Verification items for this drawing (mm, ordinates from the low corner). Give positions to 0.01 mm unless a question says otherwise; leave off trailing zeros. Loops run counter-clockwise (first coordinate to the right, second up) from the corner with the lowest first, then second, coordinate; pieces in that order, holes last. Notation, with made-up numbers: M 30.25,49.25 L 89.25,49.25 A16 ccw 89.25,70.25 Z; hole C 58.25,-30.5 d5. An arc over 180 degrees is marked long. Put each result on its own line as item: value. Start each with the question number.
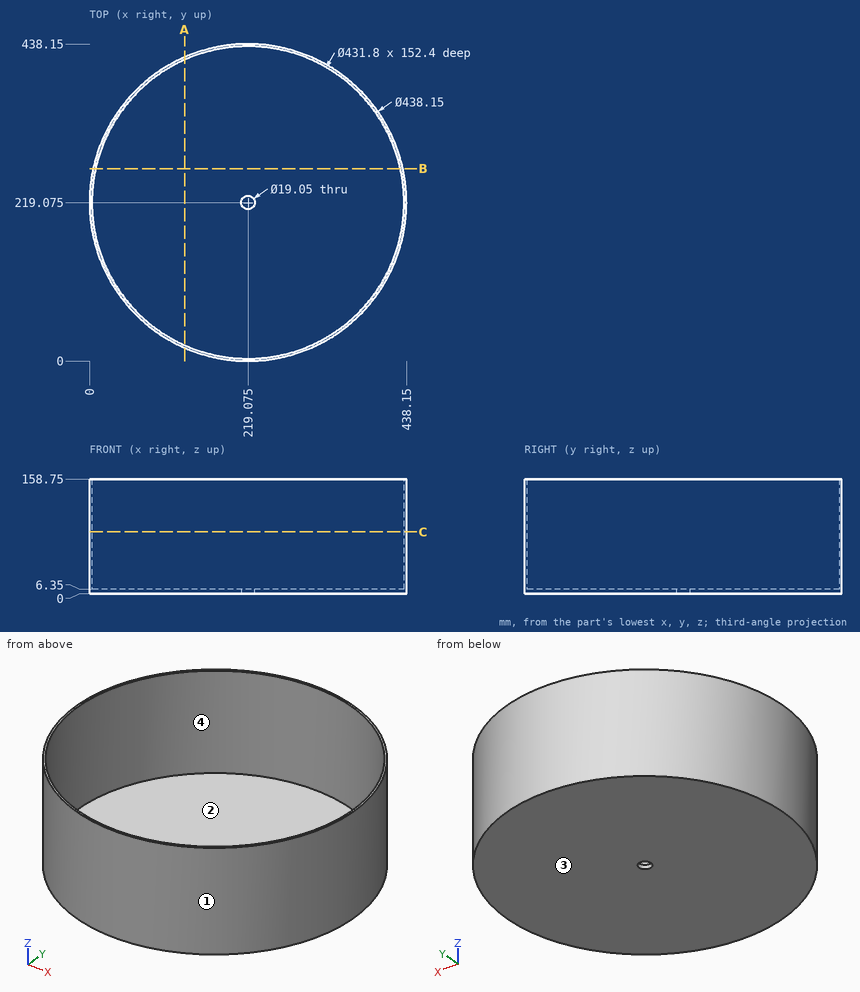
Q1. Cross-section at A-A, the plane x = 131.5. Record the boundary of the cut face in (y, z), then the cut area to 3 significant figures.
Q2. Release check for a two-part mould opening along Y. For the marked faces 1, 2, 3 and 4 record: pulls with the +Y half, pulls with the -Y half, needs draft (parallel to the pull), parting line crosses it, or undercut.
Q3. Go/stop test with flat-tipped pins: pin 1 (10 mm diameter, centred on x = 187.5, z = 50, fed in from +Y); pin 2 (8 mm diameter, centred on y = 298, z = 66.5, fed in from -X); pin 3 (1.5 mm diameter, centred on y = 169.5, z = 32, fed in from +X); pin 4 (3 mm diameter, centred on x = 224, y = 352, fed in from -Z). Record where each tip stops, or that it passes through.
Q4. Scan lines: L1, parallel to Z at x = 148, y = 392; L2, parallel to Y at x = 243.5, z = 130; L3, parallel to Y at x = 394, z = 151.5. Record each from-to range of solid material in increasing order.
Q5. Cross-section at B-B, the plane y = 266. Record the boundary of the cut face in (x, z), then the cut area to 3 significant figures.
Q6. Cross-section at C-C, the plane z = 85.5. Record the boundary of the cut face in (x, y) (3 decimals).
Ans:
1. outline: M 18.27,0 L 419.88,0 L 419.88,158.75 L 416.42,158.75 L 416.42,6.35 L 21.73,6.35 L 21.73,158.75 L 18.27,158.75 Z
1. area: 3,610 mm^2
2. face 1: parting line crosses it
2. face 2: undercut
2. face 3: needs draft
2. face 4: undercut
3. pin 1: stops at y = 436.53
3. pin 2: stops at x = 13.21
3. pin 3: stops at x = 432.64
3. pin 4: stops at z = 0
4. L1: z = 0 to 6.35
4. L2: y = 1.37 to 4.56, 433.59 to 436.78
4. L3: y = 87.18 to 92.53, 345.62 to 350.97
5. outline: M 5.08,0 L 433.07,0 L 433.07,158.75 L 429.81,158.75 L 429.81,6.35 L 8.34,6.35 L 8.34,158.75 L 5.08,158.75 Z
5. area: 3,710 mm^2
6. outline: C 219.075,219.075 d438.15; hole C 219.075,219.075 d431.8
